from build123d import *

# Parameters (mm, degrees)
F0_W     = 76.114866
F0_H     = 76.114866
F0_R     = 1.5
F0_W_2   = 3.712921
F0_H_2   = 11.138762
F0_W_3   = 41.770354
F0_H_3   = 46.411504
F0_R_2   = 1.392345
F1_DEPTH = 12


with BuildPart() as f1:
    # F0 (on Top) → F1 (new body)
    with BuildSketch(Plane.XY):
        Rectangle(F0_W, F0_H)
        with Locations((-33.557433, -33.557433)):
            Circle(F0_R, mode=Mode.SUBTRACT)
        with Locations((33.557433, -33.557433)):
            Circle(F0_R, mode=Mode.SUBTRACT)
        with Locations((-27.846902, 0)):
            Rectangle(F0_W_2, F0_H_2, mode=Mode.SUBTRACT)
        Rectangle(F0_W_3, F0_H_3, mode=Mode.SUBTRACT)
        with Locations((-33.880398, 33.880398)):
            Circle(F0_R_2, mode=Mode.SUBTRACT)
        with Locations((27.846902, 0)):
            Rectangle(F0_W_2, F0_H_2, mode=Mode.SUBTRACT)
        with Locations((33.557433, 33.557433)):
            Circle(F0_R, mode=Mode.SUBTRACT)
    extrude(amount=F1_DEPTH)


solid = f1.part
Can you work these out from the model? Positions are in its coordinate system, mm. A direction names the side the tool comes from. Give positions to 0.01 mm unless a question says otherwise; leave off trailing zeros. Order: outer loops, then holes, each group sorted by start corner. A loop starts at its lowest first (then second) coordinate and runs counter-clockwise, first axis right, second up. Notation, with made-up numbers: M 19.25,-10 L 28.25,-10 A35 ccw 28.25,25 Z; hole C 16.25,24.25 d7. An arc over 180 degrees is marked long. Use a Markdown table: item, result. Add a question column.
Item 1: Suppose I cut it at B-B (x = -17). List the corners of the cut face in (y, z) for me.
Item 2: We'd pull the mould along Y, two halves only. Please class faces 3 (the flat face through (-1, -38.057, 6)), 4 (the flat face through (-20.885, 0, 6)), 5 (the flat face through (38.057, -1, 6)): +Y half, -Y half, draft (parallel to the pull), parting line (faces both ways), or undercut.
Item 3: For faces 1 (the flat face through (-29.703, 0, 6)), 2 (the flat face through (-1, 26, 0)), which set-ups out of +Z, -Z, +X, -X, +Y, -Y let a thin tool reach every point of the face, with its end or its side?
Item 4: Suppose I cut it at D-D (z = 5.5). List the corners of the cut face in (x, y) for me.
Item 5: Suppose I cut it at C-C (y = 19). List the corners of the cut face in (x, z) for me.
Item 6: Suppose I cut it at A-A (y = -4). List the corners of the cut face in (x, z) for me, then the cut area to 3 significant figures.
Item 7: If I drill on L1, parallel to Y at x = 33.5, z = 8; L2, parallel to X at y = 4, z = 2; L3, parallel to X at y = -20.5, z = 5.5, over which ranges is the centre line in solid material (lowest first)? Write a range as [from, to].
Answer sheet:
| question | item | result |
|---|---|---|
| 1 | outline | M -38.06,0 L -23.21,0 L -23.21,12 L -38.06,12 Z; M 23.21,0 L 38.06,0 L 38.06,12 L 23.21,12 Z |
| 2 | face 3 | -Y half |
| 2 | face 4 | undercut |
| 2 | face 5 | draft |
| 3 | face 1 | +Z, -Z |
| 3 | face 2 | -Z, +X, -X, +Y, -Y |
| 4 | outline | M -38.06,-38.06 L 38.06,-38.06 L 38.06,38.06 L -38.06,38.06 Z; hole C -33.88,33.88 d2.78; hole C -33.56,-33.56 d3; hole M -29.7,-5.57 L -25.99,-5.57 L -25.99,5.57 L -29.7,5.57 Z; hole M -20.89,-23.21 L 20.89,-23.21 L 20.89,23.21 L -20.89,23.21 Z; hole M 25.99,-5.57 L 29.7,-5.57 L 29.7,5.57 L 25.99,5.57 Z; hole C 33.56,-33.56 d3; hole C 33.56,33.56 d3 |
| 5 | outline | M -38.06,0 L -20.89,0 L -20.89,12 L -38.06,12 Z; M 20.89,0 L 38.06,0 L 38.06,12 L 20.89,12 Z |
| 6 | outline | M -38.06,0 L -29.7,0 L -29.7,12 L -38.06,12 Z; M -25.99,0 L -20.89,0 L -20.89,12 L -25.99,12 Z; M 20.89,0 L 25.99,0 L 25.99,12 L 20.89,12 Z; M 29.7,0 L 38.06,0 L 38.06,12 L 29.7,12 Z |
| 6 | area | 323 mm² |
| 7 | L1 | y = [-38.06, -35.06], [-32.06, 32.06], [35.06, 38.06] |
| 7 | L2 | x = [-38.06, -29.7], [-25.99, -20.89], [20.89, 25.99], [29.7, 38.06] |
| 7 | L3 | x = [-38.06, -20.89], [20.89, 38.06] |
